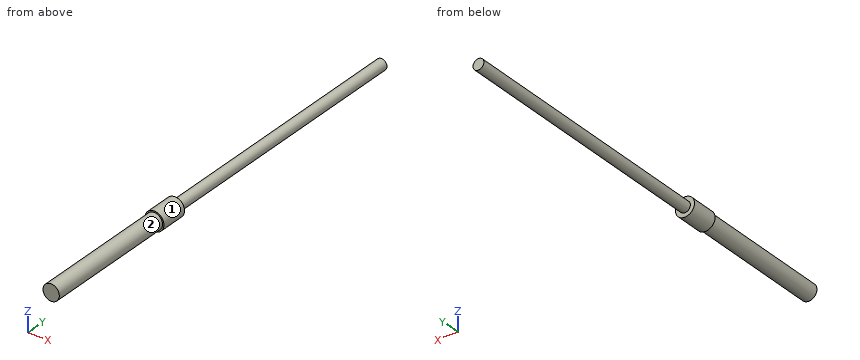
from build123d import *

# Parameters (mm, degrees)
SKETCH1_R        = 3
STEEL_TUBE_DEPTH = 50
HEATSHRINK_START = 50
SKETCH2_R        = 3.5
HEATSHRINK_DEPTH = 10
CABLE_START      = 60
SKETCH3_R        = 2
CABLE_DEPTH      = 100


with BuildPart() as part:
    # Sketch1 → Steel_Tube (new body)
    with BuildSketch(Plane(origin=(0, 0, 0), x_dir=(1, 0, 0), z_dir=(0, 1, 0))):
        with Locations(Location((0, 0, 0), (0, 0, 270))):
            Circle(SKETCH1_R)
    extrude(amount=STEEL_TUBE_DEPTH)

    # Sketch2 → Heatshrink (add)
    with BuildSketch(Plane(origin=(0, 0, 0), x_dir=(1, 0, 0), z_dir=(0, 1, 0)).offset(HEATSHRINK_START)):
        with Locations(Location((0, 0, 0), (0, 0, 270))):
            Circle(SKETCH2_R)
    extrude(amount=HEATSHRINK_DEPTH)

    # Sketch3 → Cable (add)
    with BuildSketch(Plane(origin=(0, 0, 0), x_dir=(1, 0, 0), z_dir=(0, 1, 0)).offset(CABLE_START)):
        with Locations(Location((0, 0, 0), (0, 0, 270))):
            Circle(SKETCH3_R)
    extrude(amount=CABLE_DEPTH)


solid = part.part
Here's how the part is built. I have some questions about the finished solid (model axes, mm). Face numbers are marked on the shaded views. A direction names the side the tool comes from. Round coordinates to 2 decimals unless told otherwise and drop trailing zeros. Loops run counter-clockwise (first coordinate to the right, second up) from the corner with the lowest first, then second, coordinate; pieces in that order, holes last. Notation, with made-up numbers: (-31.5, -7.75) - (-14.5, -7.75) arc R14 ccw to (-14.5, 6.25) - close; hole circle Ø3 at (-37, -26). An arc over 180 degrees is marked (long way). One line per question, with ' | ' between items. Start each with the question number.
Q1. I want a section at A-A (x = 0). Write out the boundary of the cut face in (y, z).
Q2. Please list where these lines run through material, in increasing order: line 1 (X direction, y = 147, z = -0.25); line 2 (Y direction, x = -1, z = 2.25); line 3 (Y direction, x = 3, z = -1.75). Write a range as [from, to].
Q3. Will these pins go through, and if not, where does the flat tip stop? pin 1 (3 mm diameter, centred on x = 1, y = 69.5, fed in from -Z); pin 2 (2 mm diameter, centred on y = 138, z = -0.5, fed in from -X).
Q4. I want a section at D-D (y = 40). Write out the boundary of the cut face in (x, z).
Q5. For the marked faces 1 and 2, which set-ups out of +Z, -Z, +X, -X, +Y, -Y let a thin tool reach every point of the face, with its end or its side?
Q6. I want a section at C-C (y = 72.5). Write out the boundary of the cut face in (x, z), then the cut area to 3 significant figures.
Q7. I want a section at B-B (z = 0). Write out the boundary of the cut face in (x, y).
Response values:
1) outline: (0, -3) - (50, -3) - (50, -3.5) - (60, -3.5) - (60, -2) - (160, -2) - (160, 2) - (60, 2) - (60, 3.5) - (50, 3.5) - (50, 3) - (0, 3) - close
2) line 1: x = [-1.98, 1.98] | line 2: y = [0, 60] | line 3: y = [50, 60]
3) pin 1: stops at z = -2 | pin 2: stops at x = -2
4) outline: circle Ø6 at (0, 0)
5) face 1: +Y, -Y | face 2: -Y
6) outline: circle Ø4 at (0, 0) | area: 12.6 mm²
7) outline: (-3.5, 50) - (-3, 50) - (-3, 0) - (3, 0) - (3, 50) - (3.5, 50) - (3.5, 60) - (2, 60) - (2, 160) - (-2, 160) - (-2, 60) - (-3.5, 60) - close
